```python
from build123d import *

# Parameters (mm, degrees)
F0_R          = 15.875
F1_DEPTH      = 431.8
F3_DEPTH      = 67.056
F3_DEPTH_BACK = 51.816
F6_R          = 5.08


# Not quite as in the source:
# - a feature of the source that left no trace in its solid (it failed there, or was rolled back) is left out


with BuildPart() as f1:
    # F0 (on Right) → F1 (new body)
    with BuildSketch(Plane.YZ):
        with BuildLine():
            Line((-342.5169996576, 21.7714285714), (-13.0830003424, 21.7714285714))
            ThreePointArc((-13.0830003424, 21.7714285714), (0, -25.4), (13.0830003424, 21.7714285714))
            Line((13.0830003424, 21.7714285714), (13.0830003424, 31.2964285714))
            Line((13.0830003424, 31.2964285714), (-342.5169996576, 31.2964285714))
            Line((-342.5169996576, 31.2964285714), (-342.5169996576, 24.9464285714))
            Line((-342.5169996576, 24.9464285714), (-342.5169996576, 21.7714285714))
        make_face()
        Circle(F0_R, mode=Mode.SUBTRACT)
    extrude(amount=F1_DEPTH)

    # F2 (on face) → F3 (cut, two sides)
    with BuildSketch(Plane(origin=(0, 13.0830003424, 0), x_dir=(-1, 0, 0), z_dir=(0, 1, 0))) as f3_sk:
        Polygon((-101.6, 21.7714285714), (-215.9, 21.7714285714), (-330.2, 21.7714285714), (-330.2, -30.4525513202), (-228.6, -30.4525513202), (-101.6, -30.4525513202), align=None)
    extrude(amount=-F3_DEPTH, mode=Mode.SUBTRACT)
    extrude(f3_sk.sketch, amount=F3_DEPTH_BACK, mode=Mode.SUBTRACT)

    # F5: F1 across plane


with BuildPart() as f1_1:
    add(f1.part)
    add(f1.part.mirror(Plane.XZ.offset(174.625)))

    # F6
    f6_edges = [f1_1.edges().sort_by_distance(p)[0] for p in [
        (50.8, -362.333, 21.771429),
        (381, -362.333, 21.771429),
        (50.8, 13.083, 21.771429),
        (381, 13.083, 21.771429),
    ]]
    fillet(f6_edges, radius=F6_R)


solid = f1_1.part
```
Geometry check sheet. Reference: the model listing, model coordinates, mm. A direction names the side the tool comes from. Coordinates: 2 decimals unless noted, no trailing zeros. Order: outer loops, then holes, each group sorted by start corner. A loop starts at its lowest first (then second) coordinate and runs counter-clockwise, first axis right, second up.
Item 1: Mould release check, pull along X, two halves, no side actions. Record for faces 4 (the flat face through (0, -176, 24)), 5 (the flat face through (330.2, 0, -17)), 6 (the cylindrical face through (380.29, -364.39, 4.77)), 7 (the flat face through (431.8, -176, 24)): released by +X, released by -X, zero draft, split by the parting line, or undercut.
Item 2: Section check C-C (x = 27.5). Enter the section's corners in (y, z) (3 decimals).
Item 3: Scan lines: line 1 along Y through (x, z) = (55, 0) (3 decimals); line 2 along Y through (x, z) = (35, -1); line 3 along X through (y, z) = (-25, -2.5). Record each from-to range of solid material in increasing order.
Item 4: Depth check by flat-ended pin: pin 1 (5 mm diameter, centred on x = 162, z = 28.5, fed in from +Y); pin 2 (25 mm diameter, centred on y = -2, z = 2, fed in from -X); pin 3 (8 mm diameter, centred on x = 247, y = -197.5, fed in from -Z); pin 4 (5 mm diameter, centred on x = 242, z = 29, fed in from -Y). Enter the tip coordinate at first touch or a pass-through.
Item 5: Tool access check on faces 1 (the flat face through (330.2, -350, -17)), 2 (the flat face through (213, -362.333, 28)), 3 (the flat face through (213, 13.083, 28)). Record the directions out of +Z, -Z, +X, -X, +Y, -Y that give a thin tool (end or side, any length) a straight path to the whole face; none if there is none.
Item 6: Section check B-B (z = 0). Count the separate pieces of the cut face and the enclosed holes in it, plus the area to 3 significant figures.
Item 7: Section check D-D (y = -267). Enter the section's corners in (x, z).
Item 8: Section check A-A (y = 0). Enter the section's corners in (x, z) (3 decimals), plus the area to 3 significant figures.
Check sheet entries:
1. face 4: released by -X
1. face 5: undercut
1. face 6: zero draft
1. face 7: released by +X
2. outline: (-364.386, 20.398) arc R25.4 ccw (long way) to (-336.167, 21.771) - (-13.083, 21.771) arc R25.4 ccw (long way) to (15.136, 20.398) arc R5.08 cw to (13.083, 24.477) - (13.083, 31.296) - (-362.333, 31.296) - (-362.333, 24.477) arc R5.08 cw to start; hole circle Ø31.75 at (-349.25, 0); hole circle Ø31.75 at (0, 0)
3. line 1: y = -374.65 to -365.125, -333.375 to -323.85, -25.4 to -15.875, 15.875 to 25.4
3. line 2: y = -374.63 to -365.09, -333.41 to -323.87, -25.38 to -15.84, 15.84 to 25.38
3. line 3: x = 0 to 101.6, 330.2 to 431.8
4. pin 1: stops at y = 13.08
4. pin 2: passes through
4. pin 3: stops at z = 21.77
4. pin 4: stops at y = -362.33
5. face 1: -Z, +Y, -Y
5. face 2: +Z, -Y
5. face 3: +Z, +Y
6. separate pieces: 8
6. enclosed holes: 0
6. area: 7,740 mm2
7. outline: (0, 21.77) - (431.8, 21.77) - (431.8, 31.3) - (0, 31.3) - close
8. outline: (0, -25.4) - (101.6, -25.4) - (101.6, -15.875) - (0, -15.875) - close; (0, 15.875) - (101.6, 15.875) - (101.6, 21.771) - (330.2, 21.771) - (330.2, 15.875) - (431.8, 15.875) - (431.8, 31.296) - (0, 31.296) - close; (330.2, -25.4) - (431.8, -25.4) - (431.8, -15.875) - (330.2, -15.875) - close
8. area: 7,250 mm2
